Part model, mm, in its own coordinate system. A direction names the side the tool comes from. Give positions to 0.01 mm unless a question says otherwise; leave off trailing zeros. Order: outer loops, then holes, each group sorted by start corner. A loop starts at its lowest first (then second) coordinate and runs counter-clockwise, first axis right, second up. Notation, with made-up numbers: M 75,38 L 80,38 A18 ccw 80,65 Z; hole C 74.25,14.5 d8. An arc over 180 degrees is marked long. Write each question's results on one line, items separated by ' | '. Start each with the question number.
from build123d import *

# Parameters (mm, degrees)
SKETCH1_W           = 200
SKETCH1_H           = 95
SKETCH1_R           = 1.75
BOSS_EXTRUDE1_DEPTH = 5
SKETCH2_R           = 15.75
SKETCH2_R_2         = 12.5
CUT_EXTRUDE1_DEPTH  = 5
SKETCH4_W           = 16
SKETCH4_H           = 37
BOSS_EXTRUDE2_DEPTH = 4.2
SKETCH6_W           = 20
SKETCH6_H           = 95
BOSS_EXTRUDE3_DEPTH = 3
BOSS_EXTRUDE4_START = 4
BOSS_EXTRUDE4_DEPTH = 4
SKETCH9_R           = 14
BOSS_EXTRUDE5_DEPTH = 2
CUT_EXTRUDE2_DEPTH  = 5
SKETCH11_R          = 1.75
CUT_EXTRUDE3_DEPTH  = 10
SKETCH14_R          = 1.75
SKETCH14_R_2        = 12.5
CUT_EXTRUDE4_DEPTH  = 10
CUT_EXTRUDE5_DEPTH  = 5


with BuildPart() as part:
    # Sketch1 → Boss-Extrude1 (new body)
    with BuildSketch(Plane(origin=(0, 0, 0), x_dir=(1, 0, 0), z_dir=(0, 1, 0))):
        Rectangle(SKETCH1_W, SKETCH1_H)
        with Locations(Location((-96, 43.5, 0), (0, 0, 270))):
            Circle(SKETCH1_R, mode=Mode.SUBTRACT)
        with Locations(Location((-96, -43.5, 0), (0, 0, 270))):
            Circle(SKETCH1_R, mode=Mode.SUBTRACT)
        with Locations(Location((97, 43.5, 0), (0, 0, 270))):
            Circle(SKETCH1_R, mode=Mode.SUBTRACT)
        with Locations(Location((97, -43.5, 0), (0, 0, 270))):
            Circle(SKETCH1_R, mode=Mode.SUBTRACT)
    extrude(amount=BOSS_EXTRUDE1_DEPTH)

    # Sketch2 → Cut-Extrude1 (cut)
    with BuildSketch(Plane(origin=(0, 5, 0), x_dir=(1, 0, 0), z_dir=(0, 1, 0))):
        with Locations((33, -2.5)):
            Circle(SKETCH2_R)
        with BuildLine():
            ThreePointArc((48.75, -2.5), (39.02726406, -17.051102637), (21.863068196, -13.636931804))
            Line((21.863068196, -13.636931804), (46.863068196, -38.636931804))
            ThreePointArc((46.863068196, -38.636931804), (51.97273594, -12.948897363), (73.75, -27.5))
            ThreePointArc((73.75, -27.5), (72.551102637, -33.52726406), (69.136931804, -38.636931804))
            Line((69.136931804, -38.636931804), (94.136931804, -13.636931804))
            ThreePointArc((94.136931804, -13.636931804), (67.25, -2.5), (94.136931804, 8.636931804))
            Line((94.136931804, 8.636931804), (69.136931804, 33.636931804))
            ThreePointArc((69.136931804, 33.636931804), (72.551102637, 28.52726406), (73.75, 22.5))
            ThreePointArc((73.75, 22.5), (51.97273594, 7.948897363), (46.863068196, 33.636931804))
            Line((46.863068196, 33.636931804), (21.863068196, 8.636931804))
            ThreePointArc((21.863068196, 8.636931804), (39.02726406, 12.051102637), (48.75, -2.5))
        make_face()
        with Locations((58, -27.5)):
            Circle(SKETCH2_R)
        with Locations((83, -2.5)):
            Circle(SKETCH2_R)
        with Locations((58, 22.5)):
            Circle(SKETCH2_R)
        with Locations(Location((-82, -27.5, 0), (0, 0, 270))):
            Circle(SKETCH2_R_2)
    extrude(amount=-CUT_EXTRUDE1_DEPTH, mode=Mode.SUBTRACT)

    # Sketch4 → Boss-Extrude2 (add)
    with BuildSketch(Plane.XZ):
        with Locations((-82.5, -19.5)):
            Rectangle(SKETCH4_W, SKETCH4_H)
    extrude(amount=BOSS_EXTRUDE2_DEPTH)

    # Sketch6 → Boss-Extrude3 (add)
    with BuildSketch(Plane(origin=(0, 5, 0), x_dir=(1, 0, 0), z_dir=(0, 1, 0))):
        with Locations((-110, 0)):
            Rectangle(SKETCH6_W, SKETCH6_H)
        with Locations((110, 0)):
            Rectangle(SKETCH6_W, SKETCH6_H)
    extrude(amount=-BOSS_EXTRUDE3_DEPTH)

    # Sketch8 → Boss-Extrude4 (add)
    with BuildSketch(Plane(origin=(0, 5, 0), x_dir=(1, 0, 0), z_dir=(0, 1, 0)).offset(BOSS_EXTRUDE4_START)):
        with BuildLine():
            Line((71.258252147, -40.758252147), (96.258252147, -15.758252147))
            ThreePointArc((96.258252147, -15.758252147), (101.75, -2.5), (96.258252147, 10.758252147))
            Line((96.258252147, 10.758252147), (71.258252147, 35.758252147))
            ThreePointArc((71.258252147, 35.758252147), (58, 41.25), (44.741747853, 35.758252147))
            Line((44.741747853, 35.758252147), (19.741747853, 10.758252147))
            ThreePointArc((19.741747853, 10.758252147), (14.25, -2.5), (19.741747853, -15.758252147))
            Line((19.741747853, -15.758252147), (44.741747853, -40.758252147))
            ThreePointArc((44.741747853, -40.758252147), (58, -46.25), (71.258252147, -40.758252147))
        make_face()
        with BuildLine():
            Line((21.863068196, -13.636931804), (46.863068196, -38.636931804))
            ThreePointArc((46.863068196, -38.636931804), (58, -43.25), (69.136931804, -38.636931804))
            Line((69.136931804, -38.636931804), (94.136931804, -13.636931804))
            ThreePointArc((94.136931804, -13.636931804), (98.75, -2.5), (94.136931804, 8.636931804))
            Line((94.136931804, 8.636931804), (69.136931804, 33.636931804))
            ThreePointArc((69.136931804, 33.636931804), (58, 38.25), (46.863068196, 33.636931804))
            Line((46.863068196, 33.636931804), (21.863068196, 8.636931804))
            ThreePointArc((21.863068196, 8.636931804), (17.25, -2.5), (21.863068196, -13.636931804))
        make_face(mode=Mode.SUBTRACT)
    extrude(amount=-BOSS_EXTRUDE4_DEPTH)

    # Sketch9 → Boss-Extrude5 (add)
    with BuildSketch(Plane(origin=(0, 9, 0), x_dir=(1, 0, 0), z_dir=(0, 1, 0))):
        with BuildLine():
            Line((21.863068196, -13.636931804), (46.863068196, -38.636931804))
            ThreePointArc((46.863068196, -38.636931804), (58, -43.25), (69.136931804, -38.636931804))
            Line((69.136931804, -38.636931804), (94.136931804, -13.636931804))
            ThreePointArc((94.136931804, -13.636931804), (98.75, -2.5), (94.136931804, 8.636931804))
            Line((94.136931804, 8.636931804), (69.136931804, 33.636931804))
            ThreePointArc((69.136931804, 33.636931804), (58, 38.25), (46.863068196, 33.636931804))
            Line((46.863068196, 33.636931804), (21.863068196, 8.636931804))
            ThreePointArc((21.863068196, 8.636931804), (17.25, -2.5), (21.863068196, -13.636931804))
        make_face()
        with Locations(Location((58, 22.5, 0), (0, 0, 270))):
            Circle(SKETCH9_R, mode=Mode.SUBTRACT)
        with Locations(Location((83, -2.5, 0), (0, 0, 270))):
            Circle(SKETCH9_R, mode=Mode.SUBTRACT)
        with Locations(Location((58, -27.5, 0), (0, 0, 270))):
            Circle(SKETCH9_R, mode=Mode.SUBTRACT)
        with Locations(Location((33, -2.5, 0), (0, 0, 270))):
            Circle(SKETCH9_R, mode=Mode.SUBTRACT)
    extrude(amount=-BOSS_EXTRUDE5_DEPTH)

    # Sketch10 → Cut-Extrude2 (cut)
    with BuildSketch(Plane(origin=(0, 5, 0), x_dir=(1, 0, 0), z_dir=(0, 1, 0))):
        Polygon((0, 38.5), (-7.071067812, 31.428932188), (0, 24.357864376), (7.071067812, 31.428932188), align=None)
    extrude(amount=-CUT_EXTRUDE2_DEPTH, mode=Mode.SUBTRACT)

    # Sketch11 → Cut-Extrude3 (cut)
    with BuildSketch(Plane(origin=(0, 5, 0), x_dir=(1, 0, 0), z_dir=(0, 1, 0))):
        with Locations(Location((-36.428932188, 43.5, 0), (0, 0, 270))):
            Circle(SKETCH11_R)
        with Locations(Location((-26.428932188, 43.5, 0), (0, 0, 270))):
            Circle(SKETCH11_R)
        with Locations(Location((5, -43.5, 0), (0, 0, 270))):
            Circle(SKETCH11_R)
        with Locations(Location((-5, -43.5, 0), (0, 0, 270))):
            Circle(SKETCH11_R)
    extrude(amount=-CUT_EXTRUDE3_DEPTH, mode=Mode.SUBTRACT)

    # Sketch14 → Cut-Extrude4 (cut)
    # profile 1 of 2: a face of its own
    with BuildSketch(Plane(origin=(0, 5, 0), x_dir=(1, 0, 0), z_dir=(0, 1, 0))):
        Polygon((0, 0), (-31.428932188, 31.428932188), (-31.428932188, 47.5), (-120, 47.5), (-120, -47.5), (0, -47.5), align=None)
        with Locations((-96, -43.5)):
            Circle(SKETCH14_R, mode=Mode.SUBTRACT)
        with Locations((-82, -27.5)):
            Circle(SKETCH14_R_2, mode=Mode.SUBTRACT)
        with Locations((-5, -43.5)):
            Circle(SKETCH14_R, mode=Mode.SUBTRACT)
        with Locations((-96, 43.5)):
            Circle(SKETCH14_R, mode=Mode.SUBTRACT)
        with Locations((-36.428932188, 43.5)):
            Circle(SKETCH14_R, mode=Mode.SUBTRACT)
    # profile 2 of 2: a face of its own
    with BuildSketch(Plane(origin=(0, 5, 0), x_dir=(1, 0, 0), z_dir=(0, 1, 0))):
        with Locations((-82, -27.5)):
            Circle(SKETCH14_R_2)
    extrude(amount=-CUT_EXTRUDE4_DEPTH, mode=Mode.SUBTRACT)

    # Sketch15 → Cut-Extrude5 (cut)
    with BuildSketch(Plane(origin=(0, 5, 0), x_dir=(1, 0, 0), z_dir=(0, 1, 0))):
        Polygon((-29.928932188, 47.5), (-31.428932188, 47.5), (-31.428932188, 31.428932188), (0, 0), (0, -47.5), (1.5, -47.5), (1.5, 0.621320344), (-29.928932188, 32.050252532), align=None)
    extrude(amount=-CUT_EXTRUDE5_DEPTH, mode=Mode.SUBTRACT)


solid = part.part
(1) Pull direction Z, two halves, no side cores. Call faces 1 (the flat face through (57, 9, 2)), 2 (the cylindrical face through (58.21, 7.03, -41.25)), 3 (the flat face through (3.486, 2.535, -27.844)): +Z half, -Z half, draft (parallel to the pull), parting line (faces both ways), or undercut.
(2) Saw through at D-D on z = -22.5. Give the cut face in (x, y), plus the area to 3 significant figures.
(3) Drop flat-ended pins along their axis: P1, Ø1.5, axis at y = 5, z = -7.5, coming from the -X side; P2, Ø22.5, axis at x = 83, z = 2.5, coming from the -Y side; P3, Ø4, axis at x = 97, z = -43.5, coming from the -Y side; P4, Ø4.5, axis at x = 97, z = 43.5, coming from the +Y side. Give the stop position or say it passes through.
(4) Saw through at C-C on x = 33. Give the cut face in (y, z).
(5) Tool access for faces 4 (the flat face through (83.583, 7.028, 28.433)), 5 (the flat face through (110, 2, -1)), 6 (the flat face through (81.812, 3.549, -20.962)), 7 (the cylindrical face through (14.25, 7.03, 2.29)): list every direction of +Z, -Z, +X, -X, +Y, -Y with a clear straight run to the whole face (end or side of a thin tool).
(6) Saw through at B-B on x = 58. Give the cut face in (y, z).
(7) Probe L1, parallel to X at y = 7.5, z = 1.5; L2, parallel to X at y = 1.7, z = -43.5; L3, parallel to Z at x = 24, y = 2.5. List the from-to ranges inside material, lowest first.
(8) Saw through at A-A on z = -43.5. Give the cut face in (x, y), plus the area to 3 significant figures.
Taken from the geometry:
1) face 1: draft | face 2: -Z half | face 3: undercut
2) outline: M -20.38,0 L 35.73,0 L 35.73,7 L 44,7 L 44,9 L 31.48,9 L 31.48,5 L -20.38,5 Z; M 72,7 L 80.27,7 L 80.27,0 L 100,0 L 100,2 L 120,2 L 120,5 L 84.52,5 L 84.52,9 L 72,9 Z | area: 506 mm²
3) P1: stops at x = -6.13 | P2: passes through | P3: stops at y = 0 | P4: stops at y = 5
4) outline: M 0,-47.5 L 5,-47.5 L 5,-24.02 L 9,-24.02 L 9,-11.5 L 7,-11.5 L 7,-19.77 L 0,-19.77 Z; M 0,24.77 L 7,24.77 L 7,16.5 L 9,16.5 L 9,29.02 L 5,29.02 L 5,47.5 L 0,47.5 Z
5) face 4: +Z, +X, +Y | face 5: +Z, -Z, +X, -Y | face 6: -Y | face 7: -X, +Y
6) outline: M 0,-47.5 L 5,-47.5 L 5,-41.25 L 9,-41.25 L 9,-36.5 L 7,-36.5 L 7,-38.25 L 0,-38.25 Z; M 0,43.25 L 7,43.25 L 7,41.5 L 9,41.5 L 9,46.25 L 5,46.25 L 5,47.5 L 0,47.5 Z; M 7,-8.5 L 9,-8.5 L 9,13.5 L 7,13.5 Z
7) L1: x = 14.28 to 19.04, 46.96 to 69.04, 96.96 to 101.72 | L2: x = -29.93 to -28.18, -24.68 to 95.25, 98.75 to 100 | L3: z = -47.5 to -10.77, 15.77 to 47.5
8) outline: M -29.93,0 L -28.18,0 L -28.18,5 L -29.93,5 Z; M -24.68,0 L 95.25,0 L 95.25,5 L -24.68,5 Z; M 98.75,0 L 100,0 L 100,2 L 120,2 L 120,5 L 98.75,5 Z | area: 675 mm²
